```python
from build123d import *

# Parameters (mm, degrees)
SKETCH1_W           = 306.04968
SKETCH1_H           = 215.9
SKETCH1_W_2         = 255.24968
SKETCH1_H_2         = 165.1
BOSS_EXTRUDE1_DEPTH = 25.4
SKETCH10_W          = 306.04968
SKETCH10_H          = 139.69956566
SKETCH10_W_2        = 255.24968
SKETCH10_H_2        = 88.89956566
BOSS_EXTRUDE6_DEPTH = 12.7
SKETCH12_W          = 25.328039302
SKETCH12_H          = 139.69956566
BOSS_EXTRUDE7_DEPTH = 15.30096
SKETCH14_W          = 60.96
SKETCH14_H          = 60.96
CUT_EXTRUDE1_DEPTH  = 195.734349014
SKETCH5_W           = 25.4
SKETCH5_H           = 215.9
BOSS_EXTRUDE4_DEPTH = 38.1


with BuildPart() as part:
    # Sketch1 → Boss-Extrude1 (new body)
    # profile 1 of 2: a face of its own
    with BuildSketch(Plane.XY):
        Rectangle(SKETCH1_W, SKETCH1_H)
        Rectangle(SKETCH1_W_2, SKETCH1_H_2, mode=Mode.SUBTRACT)
    # profile 2 of 2: a face of its own
    with BuildSketch(Plane.XY):
        Rectangle(SKETCH1_W_2, SKETCH1_H_2)
    extrude(amount=BOSS_EXTRUDE1_DEPTH)

    # Sketch10 → Boss-Extrude6 (add)
    with BuildSketch(Plane.XY.offset(25.4)):
        Rectangle(SKETCH10_W, SKETCH10_H)
        Rectangle(SKETCH10_W_2, SKETCH10_H_2, mode=Mode.SUBTRACT)
    extrude(amount=BOSS_EXTRUDE6_DEPTH)

    # Sketch12 → Boss-Extrude7 (add)
    with BuildSketch(Plane.XY.offset(38.1)):
        with Locations((140.360820349, 0)):
            Rectangle(SKETCH12_W, SKETCH12_H)
    extrude(amount=BOSS_EXTRUDE7_DEPTH)

    # Sketch14 → Cut-Extrude1 (cut, through all)
    with BuildSketch(Plane(origin=(0, 0, 0), x_dir=(-1, 0, 0), z_dir=(0, 0, -1))):
        with Locations((0, 38.1)):
            Rectangle(SKETCH14_W, SKETCH14_H)
    extrude(amount=-CUT_EXTRUDE1_DEPTH, mode=Mode.SUBTRACT)

    # Sketch5 → Boss-Extrude4 (add)
    with BuildSketch(Plane.ZY.offset(153.02484)):
        with Locations((12.7, 0)):
            Rectangle(SKETCH5_W, SKETCH5_H)
    extrude(amount=BOSS_EXTRUDE4_DEPTH)


solid = part.part
```
Work out the finished part from the listing and answer in its coordinate system (mm). A direction names the side the tool comes from. Give positions to 0.01 mm unless a question says otherwise; leave off trailing zeros. Write each loop counter-clockwise with the first axis right and the second up, starting at its lowest first coordinate (ties: lowest second). Pieces come first, ordered by that corner, then holes.
(1) Straight lines are drawn through the part: line 1 (Y direction, x = -69.5, z = 31); line 2 (Y direction, x = 29, z = 38); line 3 (X direction, y = 61, z = 22). For each, find the intervals that lie inside material, in ascending order.
Final values:
line 1: y = -69.85 to -44.45, 44.45 to 69.85
line 2: y = -69.85 to -44.45, 68.58 to 69.85
line 3: x = -191.12 to -30.48, 30.48 to 153.02
(2) The part is cut by section D-D on y = -63.5. Write down the section's boundary in (x, z), plus the area to 3 significant figures.
Final values:
outline: (-191.12, 0) - (153.02, 0) - (153.02, 53.4) - (127.7, 53.4) - (127.7, 38.1) - (-153.02, 38.1) - (-153.02, 25.4) - (-191.12, 25.4) - close
area: 13,000 mm2
(3) The mould has two halves that part along Y. Classify faces 1 (the flat face through (-2, -44.45, 32)), 2 (the flat face through (-2, 69.85, 33)), 3 (the flat face through (-153.025, -1, 32)): pulls with the +Y half, pulls with the -Y half, needs draft (parallel to the pull), parting line crosses it, or undercut.
Final values:
face 1: undercut
face 2: pulls with the +Y half
face 3: needs draft
(4) Flat-ended cylindrical pins translate along their axes: pin 1 Ø4 at (y, z) = (66.5, 41.5) entering from -X; pin 2 Ø1 at (y, z) = (-33.5, 36.5) entering from -X; pin 3 Ø1.5 at (x, y) = (-95.5, 36) entering from -Z; pin 4 Ø14 at (x, z) = (81.5, 33.5) entering from -Y. Find the tip coordinate at first contact, or state that the pin passes through.
Final values:
pin 1: stops at x = 127.7
pin 2: stops at x = -153.02
pin 3: stops at z = 0
pin 4: stops at y = -69.85
(5) Which of the six approach directions +Z, -Z, +X, -X, +Y, -Y give full straight-line access (tool end or side, diameter ignored) to faces 4 (the flat face through (-46, -46, 38.1)), 5 (the flat face through (-2, 1, 25.4)), 6 (the flat face through (153.025, -2, 20)), 7 (the flat face through (0, 68.58, 19)), 8 (the flat face through (-191.125, 2, 13))?
Final values:
face 4: +Z, -X, +Y, -Y
face 5: +Z
face 6: +Z, -Z, +X, +Y, -Y
face 7: +Z, -Z
face 8: +Z, -Z, -X, +Y, -Y
(6) The part is cut by section B-B on x = 14.5. Write down the section's boundary in (y, z).
Final values:
outline: (-107.95, 0) - (7.62, 0) - (7.62, 25.4) - (-44.45, 25.4) - (-44.45, 38.1) - (-69.85, 38.1) - (-69.85, 25.4) - (-107.95, 25.4) - close; (68.58, 0) - (107.95, 0) - (107.95, 25.4) - (69.85, 25.4) - (69.85, 38.1) - (68.58, 38.1) - close
(7) The part is cut by section C-C on z = 20. Write down the section's boundary in (x, y), plus the area to 3 significant figures.
Final values:
outline: (-191.12, -107.95) - (153.02, -107.95) - (153.02, 107.95) - (-191.12, 107.95) - close; hole (-30.48, 7.62) - (30.48, 7.62) - (30.48, 68.58) - (-30.48, 68.58) - close
area: 70,600 mm2
(8) The part is cut by section A-A on y = 33. Write down the section's boundary in (x, z).
Final values:
outline: (-191.12, 0) - (-30.48, 0) - (-30.48, 25.4) - (-127.62, 25.4) - (-127.62, 38.1) - (-153.02, 38.1) - (-153.02, 25.4) - (-191.12, 25.4) - close; (30.48, 0) - (153.02, 0) - (153.02, 53.4) - (127.7, 53.4) - (127.7, 38.1) - (127.62, 38.1) - (127.62, 25.4) - (30.48, 25.4) - close
